Job drawing, mm, ordinate dimensions from the low corner. One solid piece. Coordinates: 2 decimals unless noted, no trailing zeros. Write each loop counter-clockwise with the first axis right and the second up, starting at its lowest first coordinate (ties: lowest second). Pieces come first, ordered by that corner, then holes.
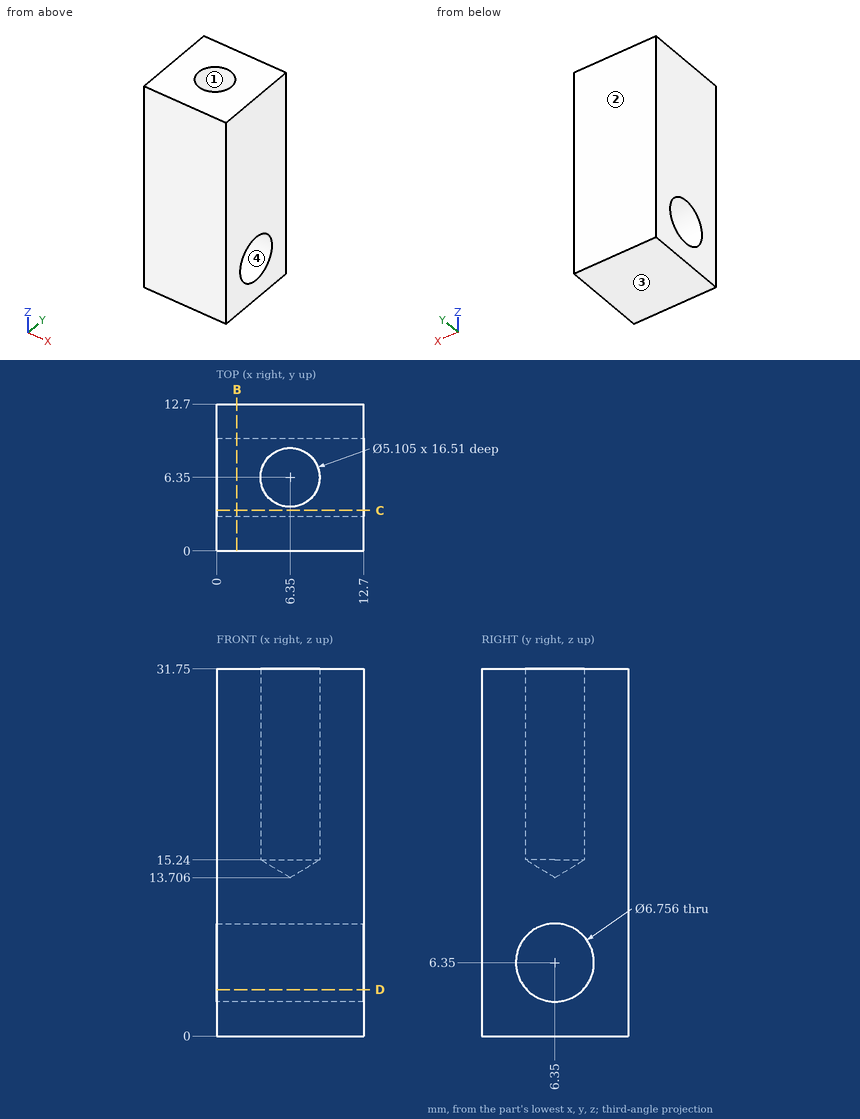
1. Saw through at C-C on y = 3.5. List the corners of the cut face in (x, z).
Computed values:
outline: (0, 0) - (12.7, 0) - (12.7, 4.54) - (0, 4.54) - close; (0, 8.16) - (12.7, 8.16) - (12.7, 31.75) - (0, 31.75) - close
2. Probe line 1 along X through (y, z) = (6.5, 16); line 2 along Y through (x, z) = (6, 6.35). List the from-to ranges inside material, lowest first.
Computed values:
line 1: x = 0 to 3.8, 8.9 to 12.7
line 2: y = 0 to 2.97, 9.73 to 12.7
3. Saw through at B-B on x = 1.75. List the corners of the cut face in (y, z).
Computed values:
outline: (0, 0) - (12.7, 0) - (12.7, 31.75) - (0, 31.75) - close; hole circle Ø6.76 at (6.35, 6.35)
4. Mould opens along Y. For the marked faces 1, 2, 3 and 4 say: +Y half, -Y half, draft (parallel to the pull), parting line (faces both ways), or undercut.
Computed values:
face 1: undercut
face 2: +Y half
face 3: draft
face 4: undercut
5. Saw through at D-D on z = 4. List the corners of the cut face in (x, y).
Computed values:
outline: (0, 0) - (12.7, 0) - (12.7, 3.92) - (0, 3.92) - close; (0, 8.78) - (12.7, 8.78) - (12.7, 12.7) - (0, 12.7) - close
